from build123d import *

# Parameters (mm, degrees)
F0_R     = 1.477487
F0_R_2   = 1.471046
F1_DEPTH = 15


with BuildPart() as f1:
    # F0 (on Top) → F1 (new body)
    with BuildSketch(Plane.XY):
        with BuildLine():
            Line((0, 2), (0, 0))
            Line((0, 0), (39.5, 0))
            ThreePointArc((39.5, 0), (39.853553, -0.146447), (40, -0.5))
            Line((40, -0.5), (40, -9.135922))
            ThreePointArc((40, -9.135922), (39.776556, -9.552475), (39.305934, -9.596724))
            ThreePointArc((39.305934, -9.596724), (34.949923, -12.826281), (39.87787, -15.089068))
            ThreePointArc((39.87787, -15.089068), (40.013491, -15.022786), (40.162713, -15))
            Line((40.162713, -15), (45, -15))
            Line((45, -15), (47, -15))
            ThreePointArc((47, -15), (48.767767, -14.267767), (49.5, -12.5))
            Line((49.5, -12.5), (49.5, -10))
            ThreePointArc((49.5, -10), (49.25, -9.75), (49, -10))
            ThreePointArc((49, -10), (45, -14), (41, -10))
            Line((41, -10), (41, -2.565671))
            Line((41, -2.565671), (41, -0.5))
            ThreePointArc((41, -0.5), (40.267767, 1.267767), (38.5, 2))
            Line((38.5, 2), (0, 2))
        make_face()
        with Locations((38.083223, -12.5)):
            Circle(F0_R, mode=Mode.SUBTRACT)
        with BuildLine():
            Line((-39.5, 0), (0, 0))
            Line((0, 0), (0, 2))
            Line((0, 2), (-38.5, 2))
            ThreePointArc((-38.5, 2), (-40.267767, 1.267767), (-41, -0.5))
            Line((-41, -0.5), (-41, -15))
            Line((-41, -15), (-40.162713, -15))
            ThreePointArc((-40.162713, -15), (-40.013491, -15.022786), (-39.87787, -15.089068))
            ThreePointArc((-39.87787, -15.089068), (-34.949923, -12.826281), (-39.305934, -9.596724))
            ThreePointArc((-39.305934, -9.596724), (-39.776556, -9.552475), (-40, -9.135922))
            Line((-40, -9.135922), (-40, -0.5))
            ThreePointArc((-40, -0.5), (-39.853553, -0.146447), (-39.5, 0))
        make_face()
        with Locations((-38.083223, -12.5)):
            Circle(F0_R_2, mode=Mode.SUBTRACT)
    extrude(amount=F1_DEPTH)


solid = f1.part
Can you work these out from the model? Positions are in its coordinate system, mm. A direction names the side the tool comes from. Give positions to 0.01 mm unless a question says otherwise; leave off trailing zeros. Loops run counter-clockwise (first coordinate to the right, second up) from the corner with the lowest first, then second, coordinate; pieces in that order, holes last. Notation, with made-up numbers: (77.5, 29.5) -> (130.5, 29.5) arc R31 ccw to (130.5, 62.5) -> close; hole circle Ø5 at (39.25, -6). An arc over 180 degrees is marked (long way). Use one line per item in the form item = value.
1) If we section it at B-B (z = 3.5): Please give me the cut outline in (x, y), plus the area to 3 significant figures.
Answers:
outline = (-41, -15) -> (-40.16, -15) arc R0.5 cw to (-39.88, -15.09) arc R3.15 ccw (long way) to (-39.31, -9.6) arc R0.5 cw to (-40, -9.14) -> (-40, -0.5) arc R0.5 cw to (-39.5, 0) -> (39.5, 0) arc R0.5 cw to (40, -0.5) -> (40, -9.14) arc R0.5 cw to (39.31, -9.6) arc R3.15 ccw (long way) to (39.88, -15.09) arc R0.5 cw to (40.16, -15) -> (47, -15) arc R2.5 ccw to (49.5, -12.5) -> (49.5, -10) arc R0.25 ccw to (49, -10) arc R4 cw to (41, -10) -> (41, -0.5) arc R2.5 ccw to (38.5, 2) -> (-38.5, 2) arc R2.5 ccw to (-41, -0.5) -> close; hole circle Ø2.94 at (-38.08, -12.5); hole circle Ø2.95 at (38.08, -12.5)
area = 248 mm²
2) For faces 1 (the face through (40.287, 1.248, 7.395)), 2 (the face through (40, -5, 7)), which set-ups out of +Z, -Z, +X, -X, +Y, -Y let a thin tool reach every point of the face, with its end or its side?
Answers:
face_1 = +Z, -Z, +X, +Y
face_2 = +Z, -Z
3) If we section it at A-A (y = -2.5): Please give me the cut outline in (x, z).
Answers:
outline = (-41, 0) -> (-40, 0) -> (-40, 15) -> (-41, 15) -> close; (40, 0) -> (41, 0) -> (41, 15) -> (40, 15) -> close
4) If we section it at D-D (x = 30.5): Please give me the cut outline in (y, z), plus the area to 3 significant figures.
Answers:
outline = (0, 0) -> (2, 0) -> (2, 15) -> (0, 15) -> close
area = 30.0 mm²
5) Will these pins go through, and if not, where does the flat tip stop? pin 1 (5.5 mm diameter, centred on x = 43.5, z = 6.5, fed in from -Y); pin 2 (4 mm diameter, centred on y = -3, z = 9.5, fed in from +X); pin 3 (7.5 mm diameter, centred on x = 8, z = 7, fed in from -Y).
Answers:
pin_1 = -15
pin_2 = 41
pin_3 = 0
6) If we section it at C-C (x = 45): Please give me the cut outline in (y, z).
Answers:
outline = (-15, 0) -> (-14, 0) -> (-14, 15) -> (-15, 15) -> close
7) I need wall thicknesses on line 1 along X through (y, z) = (-2.75, 7.25); line 2 along X through (y, z) = (-11.75, 13.5); line 3 along Y through (x, z) = (-33, 7.25). Which ranges of each line are inside material? Lowest first, please.
Answers:
line_1 = -41 to -40, 40 to 41
line_2 = -41 to -39.35, -36.82 to -35.02, 35.02 to 36.81, 39.36 to 41.4, 48.6 to 49.5
line_3 = 0 to 2
8) We'd pull the mould along Y, two halves only. Please class faces 3 (the face through (-40.248, 1.287, 7.395)), 4 (the face through (44, -15, 7)), 5 (the face through (36.607, -12.435, 7.395)), 6 (the face through (4, 0.4, 0)): released by +Y, released by -Y, zero draft, split by the parting line, or undercut.
Answers:
face_3 = released by +Y
face_4 = released by -Y
face_5 = undercut
face_6 = zero draft
